Can you work these out from the model? Positions are in its coordinate system, mm. Face numbers are marked on the shaded views. A direction names the side the tool comes from. Round coordinates to 2 decimals unless told otherwise and drop trailing zeros. Write each loop counter-clockwise with the first axis right and the second up, starting at its lowest first coordinate (ties: lowest second). Pieces come first, ordered by that corner, then holes. Notation, with made-up numbers: (41.5, 5.5) -> (54.5, 5.5) arc R23 ccw to (54.5, 38.5) -> close; hole circle Ø7 at (31.25, 77). An arc over 180 degrees is marked (long way). Write item = value, one per line. Start each with the question number.
1) If I drill on line 1 (Y direction, x = -13.75, z = 3.15); line 2 (Y direction, x = 6, z = 2.25); line 3 (X direction, y = 12.5, z = 2.25), over which ranges is the centre line in solid material (lowest first)?
2) Imagine slicing it at B-B, the plane x = -28.75. Please give me the cut outline in (y, z).
3) Imagine slicing it at C-C, the plane y = -28.75. Please give me the cut outline in (x, z).
4) I'm going to push flat-ended pins straight in: pin 1 (16 mm diameter, centred on x = -48, y = 39, fed in from -Z); pin 2 (1.1 mm diameter, centred on x = 22.5, z = 9.5, fed in from -Y); pin 3 (16 mm diameter, centred on x = -43.75, y = 13.75, fed in from +Z); pin 4 (6 mm diameter, centred on x = 9.5, y = -42.5, fed in from -Z). Where does each tip first touch, or does it pass through?
5) Imagine slicing it at A-A, the plane y = 28.75. State how many separate pieces and enclosed holes the cut face has, then the cut area to 3 significant figures.
6) Thinking about a two-plate mould opening in Y: for the marked faces 3 and 4, which applies, +Y half, -Y half, draft (parallel to the pull), parting line (faces both ways), or undercut?
7) For the marked faces 1 and 2, which set-ups out of +Z, -Z, +X, -X, +Y, -Y let a thin tool reach every point of the face, with its end or its side?
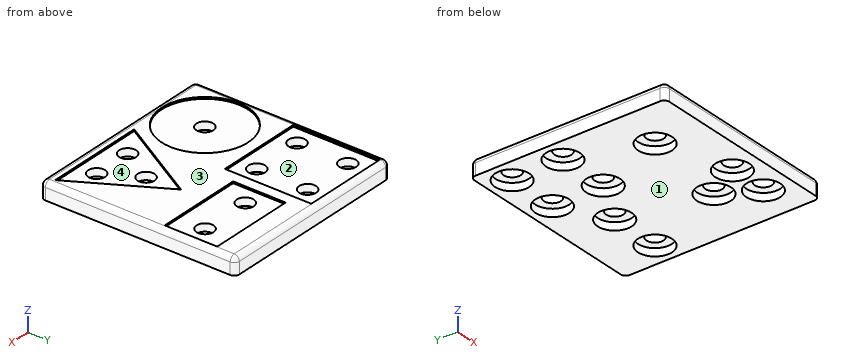
from build123d import *

# Parameters (mm, degrees)
SKETCH1_W           = 115
SKETCH1_H           = 115
BOSS_EXTRUDE1_DEPTH = 10
SKETCH2_W           = 51
SKETCH2_H           = 51
CUT_EXTRUDE1_DEPTH  = 1
SKETCH4_W           = 51
SKETCH4_H           = 31
CUT_EXTRUDE2_DEPTH  = 1
SKETCH11_R          = 25.5
SKETCH11_R_2        = 5
CUT_EXTRUDE8_DEPTH  = 1
SKETCH6_R           = 5
CUT_EXTRUDE9_DEPTH  = 1
SKETCH3_R           = 5
CUT_EXTRUDE10_DEPTH = 10
SKETCH5_R           = 5
CUT_EXTRUDE11_DEPTH = 10
SKETCH19_R          = 5
CUT_EXTRUDE12_DEPTH = 10
SKETCH20_R          = 5
CUT_EXTRUDE13_DEPTH = 10
SKETCH21_R          = 10
CUT_EXTRUDE14_DEPTH = 4.5
FILLET2_R           = 3


with BuildPart() as part:
    # Sketch1 → Boss-Extrude1 (new body)
    with BuildSketch(Plane.XY):
        Rectangle(SKETCH1_W, SKETCH1_H)
    extrude(amount=BOSS_EXTRUDE1_DEPTH)

    # Sketch2 → Cut-Extrude1 (cut)
    with BuildSketch(Plane.XY.offset(10)):
        with Locations((-28.75, 28.75)):
            Rectangle(SKETCH2_W, SKETCH2_H)
    extrude(amount=-CUT_EXTRUDE1_DEPTH, mode=Mode.SUBTRACT)

    # Sketch4 → Cut-Extrude2 (cut)
    with BuildSketch(Plane.XY.offset(10)):
        with Locations((28.75, 28.75)):
            Rectangle(SKETCH4_W, SKETCH4_H)
    extrude(amount=-CUT_EXTRUDE2_DEPTH, mode=Mode.SUBTRACT)

    # Sketch11 → Cut-Extrude8 (cut)
    with BuildSketch(Plane.XY.offset(10)):
        with Locations((-28.75, -28.75)):
            Circle(SKETCH11_R)
        with Locations((-28.75, -28.75)):
            Circle(SKETCH11_R_2, mode=Mode.SUBTRACT)
    extrude(amount=-CUT_EXTRUDE8_DEPTH, mode=Mode.SUBTRACT)

    # Sketch6 → Cut-Extrude9 (cut)
    with BuildSketch(Plane.XY.offset(10)):
        Polygon((24, -1), (-5.444863729, -52), (53.444863729, -52), align=None)
        with Locations((24, -21.666666667)):
            Circle(SKETCH6_R, mode=Mode.SUBTRACT)
        with Locations((35.547005384, -41.666666667)):
            Circle(SKETCH6_R, mode=Mode.SUBTRACT)
        with Locations((12.452994616, -41.666666667)):
            Circle(SKETCH6_R, mode=Mode.SUBTRACT)
    extrude(amount=-CUT_EXTRUDE9_DEPTH, mode=Mode.SUBTRACT)

    # Sketch3 → Cut-Extrude10 (cut)
    with BuildSketch(Plane.XY.offset(9)):
        with Locations((-43.75, 43.75)):
            Circle(SKETCH3_R)
        with Locations((-13.75, 43.75)):
            Circle(SKETCH3_R)
        with Locations((-13.75, 13.75)):
            Circle(SKETCH3_R)
        with Locations((-43.75, 13.75)):
            Circle(SKETCH3_R)
    extrude(amount=-CUT_EXTRUDE10_DEPTH, mode=Mode.SUBTRACT)

    # Sketch5 → Cut-Extrude11 (cut)
    with BuildSketch(Plane.XY.offset(9)):
        with Locations((13.75, 28.75)):
            Circle(SKETCH5_R)
        with Locations((43.75, 28.75)):
            Circle(SKETCH5_R)
    extrude(amount=-CUT_EXTRUDE11_DEPTH, mode=Mode.SUBTRACT)

    # Sketch19 → Cut-Extrude12 (cut)
    with BuildSketch(Plane.XY.offset(10)):
        with Locations((-28.75, -28.75)):
            Circle(SKETCH19_R)
    extrude(amount=-CUT_EXTRUDE12_DEPTH, mode=Mode.SUBTRACT)

    # Sketch20 → Cut-Extrude13 (cut)
    with BuildSketch(Plane.XY.offset(10)):
        with Locations((24, -21.666666667)):
            Circle(SKETCH20_R)
        with Locations((35.547005384, -41.666666667)):
            Circle(SKETCH20_R)
        with Locations((12.452994616, -41.666666667)):
            Circle(SKETCH20_R)
    extrude(amount=-CUT_EXTRUDE13_DEPTH, mode=Mode.SUBTRACT)

    # Sketch21 → Cut-Extrude14 (cut)
    with BuildSketch(Plane(origin=(0, 0, 0), x_dir=(-1, 0, 0), z_dir=(0, 0, -1))):
        with Locations((-43.75, 28.75)):
            Circle(SKETCH21_R)
        with Locations((-13.75, 28.75)):
            Circle(SKETCH21_R)
        with Locations((13.75, 43.75)):
            Circle(SKETCH21_R)
        with Locations((43.75, 43.75)):
            Circle(SKETCH21_R)
        with Locations((43.75, 13.75)):
            Circle(SKETCH21_R)
        with Locations((13.75, 13.75)):
            Circle(SKETCH21_R)
        with Locations((-24, -21.666666667)):
            Circle(SKETCH21_R)
        with Locations((28.75, -28.75)):
            Circle(SKETCH21_R)
        with Locations((-12.452994616, -41.666666667)):
            Circle(SKETCH21_R)
        with Locations((-35.547005384, -41.666666667)):
            Circle(SKETCH21_R)
    extrude(amount=-CUT_EXTRUDE14_DEPTH, mode=Mode.SUBTRACT)

    # Fillet2
    fillet2_edges = [part.edges().sort_by_distance(p)[0] for p in [
        (57.5, 0, 10),
        (0, 57.5, 10),
        (-57.5, 0, 10),
        (0, -57.5, 10),
        (-57.5, 57.5, 5),
        (57.5, 57.5, 5),
        (57.5, -57.5, 5),
        (-57.5, -57.5, 5),
    ]]
    fillet(fillet2_edges, radius=FILLET2_R)


solid = part.part
Reported:
q1.line_1 = -57.5 to 3.75, 23.75 to 33.75, 53.75 to 57.5
q1.line_2 = -57.5 to -49.31, -34.03 to 22.43, 35.07 to 57.5
q1.line_3 = -57.5 to -53.67, -33.83 to -23.67, -3.83 to 57.5
q2.outline = (-57.5, 0) -> (-38.75, 0) -> (-38.75, 4.5) -> (-33.75, 4.5) -> (-33.75, 9) -> (-54.25, 9) -> (-54.25, 10) -> (-54.5, 10) arc R3 ccw to (-57.5, 7) -> close; (-23.75, 4.5) -> (-18.75, 4.5) -> (-18.75, 0) -> (57.5, 0) -> (57.5, 7) arc R3 ccw to (54.5, 10) -> (54.25, 10) -> (54.25, 9) -> (3.25, 9) -> (3.25, 10) -> (-3.25, 10) -> (-3.25, 9) -> (-23.75, 9) -> close
q3.outline = (-57.5, 0) -> (-38.75, 0) -> (-38.75, 4.5) -> (-33.75, 4.5) -> (-33.75, 9) -> (-54.25, 9) -> (-54.25, 10) -> (-54.5, 10) arc R3 ccw to (-57.5, 7) -> close; (-23.75, 4.5) -> (-18.75, 4.5) -> (-18.75, 0) -> (16.94, 0) -> (16.94, 4.5) -> (31.06, 4.5) -> (31.06, 0) -> (57.5, 0) -> (57.5, 7) arc R3 ccw to (54.5, 10) -> (40.02, 10) -> (40.02, 9) -> (7.98, 9) -> (7.98, 10) -> (-3.25, 10) -> (-3.25, 9) -> (-23.75, 9) -> close
q4.pin_1 = 0
q4.pin_2 = -56.78
q4.pin_3 = 9
q4.pin_4 = 4.5
q5.separate_pieces = 3
q5.enclosed_holes = 0
q5.area = 774 mm²
q6.face_3 = draft
q6.face_4 = undercut
q7.face_1 = -Z, +X, -X, +Y, -Y
q7.face_2 = +Z
